For this review, use the dimensioned drawing (mm, ordinates from the lowest corner) and the shaded views. A direction names the side the tool comes from. Give positions to 0.01 mm unless a question says otherwise; leave off trailing zeros. Order: outer loops, then holes, each group sorted by start corner. A loop starts at its lowest first (then second) coordinate and runs counter-clockwise, first axis right, second up. Notation, with made-up numbers: M 1,63.5 L 27,63.5 A26 cw 27,81.5 Z; hole C 56,68 d6. An arc over 180 degrees is marked long. Use CSV: the item, a comma, the result in double quotes. Start each with the question number.
(1) Clearance check with flat-ended pins moving along their axes: P1, Ø5, axis at x = 31, y = 21, coming from the -Z side; P2, Ø8, axis at y = 14, z = 115.5, coming from the +X side; P3, Ø6, axis at y = 63, z = 40, coming from the +X side. State where each tip first meets the part, or that it passes through.
(2) Wall thickness on L1, parallel to Y at x = 37, z = 51; L2, parallel to X at y = 29, z = 52; L3, parallel to Y at x = 50, z = 133: over which ranges is each line inside the solid? List them lowest first. Write a range as from..to.
(3) Consider section A-A (x = 38.1). Write out the cut boundary in (y, z).
(4) Tool access review of the marked faces 1 and 2: name each direction out of +Z, -Z, +X, -X, +Y, -Y from which nothing blocks a thin tool from reaching the whole face with its end or side.
(5) Consider section B-B (z = 27.5). Write out the cut boundary in (x, y).
(6) Consider section C-C (z = 106). Write out the cut boundary in (x, y), and give its area (3 significant figures).
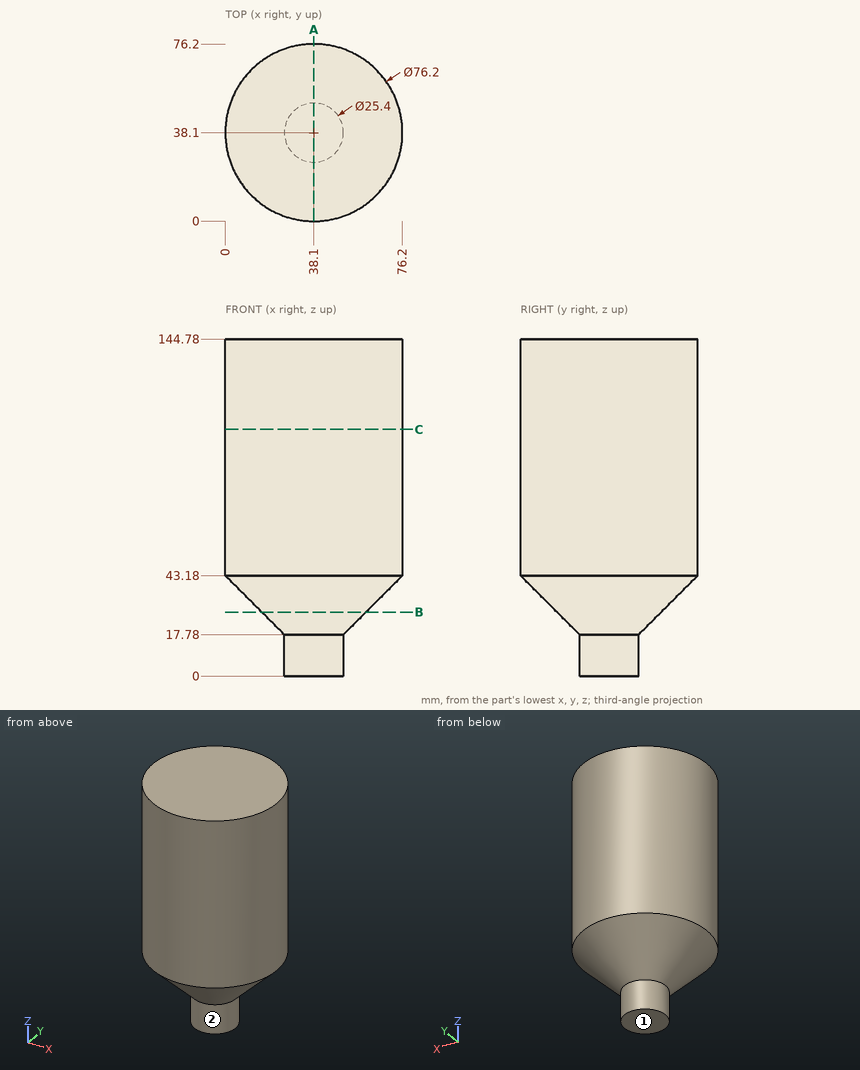
Check result:
1,P1,"stops at z = 21.1"
1,P2,"stops at x = 70.47"
1,P3,"stops at x = 67.43"
2,L1,"y = 0.02..76.18"
2,L2,"x = 1.1..75.1"
2,L3,"y = 1.91..74.29"
3,outline,"M 0,43.18 L 25.4,17.78 L 25.4,0 L 50.8,0 L 50.8,17.78 L 76.2,43.18 L 76.2,144.78 L 0,144.78 Z"
4,face 1,"-Z, +X, -X, +Y, -Y"
4,face 2,"-Z"
5,outline,"C 38.1,38.1 d44.84"
6,outline,"C 38.1,38.1 d76.2"
6,area,"4,560 mm^2"
